Check sheet for the modelled part. Datum: model origin and axes. Units: mm. Face numbers are marked on the shaded views. A direction names the side the tool comes from. Round coordinates to 2 decimals unless told otherwise and drop trailing zeros. Write each loop counter-clockwise with the first axis right and the second up, starting at its lowest first coordinate (ties: lowest second). Pieces come first, ordered by that corner, then holes. Notation, with made-up numbers: (37.25, 59.25) -> (51.25, 59.25) arc R16 ccw to (51.25, 73.25) -> close; hole circle Ø9 at (-35, 39.25). An arc over 180 degrees is marked (long way). One line per item, written item: value.
from build123d import *

# Parameters (mm, degrees)
SKETCH1_W           = 38
SKETCH1_H           = 13
BOSS_EXTRUDE1_DEPTH = 65
SKETCH2_R           = 1.848381342
SKETCH2_R_2         = 4
SKETCH2_R_3         = 1.991530231
BOSS_EXTRUDE4_DEPTH = 22
SKETCH3_R           = 1.118624503
BOSS_EXTRUDE5_DEPTH = 15


with BuildPart() as part:
    # Sketch1 → Boss-Extrude1 (new body)
    with BuildSketch(Plane(origin=(0, 0, 0), x_dir=(0, 0, -1), z_dir=(1, 0, 0))):
        Rectangle(SKETCH1_W, SKETCH1_H)
    extrude(amount=BOSS_EXTRUDE1_DEPTH)

    # Sketch2 → Boss-Extrude4 (add)
    with BuildSketch(Plane(origin=(65, 0, 0), x_dir=(0, 0, -1), z_dir=(1, 0, 0))):
        with Locations(Location((-16.455259224, -3.564649458, 0), (0, 0, 180))):
            Circle(SKETCH2_R)
        with Locations(Location((-8.1, -2.100713402, 0), (0, 0, 180))):
            Circle(SKETCH2_R_2)
        with Locations(Location((0, -2.100713402, 0), (0, 0, 180))):
            Circle(SKETCH2_R_2)
        with Locations(Location((8.1, -2.100713402, 0), (0, 0, 180))):
            Circle(SKETCH2_R_2)
        with Locations(Location((16.444267151, -3.564649458, 0), (0, 0, 180))):
            Circle(SKETCH2_R_3)
    extrude(amount=BOSS_EXTRUDE4_DEPTH)

    # Sketch3 → Boss-Extrude5 (add)
    with BuildSketch(Plane.ZY):
        with Locations((-10.926639498, -2.758613366)):
            Circle(SKETCH3_R)
        with Locations((0, -2.758613366)):
            Circle(SKETCH3_R)
        with Locations((12.420208926, -2.758613366)):
            Circle(SKETCH3_R)
    extrude(amount=BOSS_EXTRUDE5_DEPTH)


solid = part.part
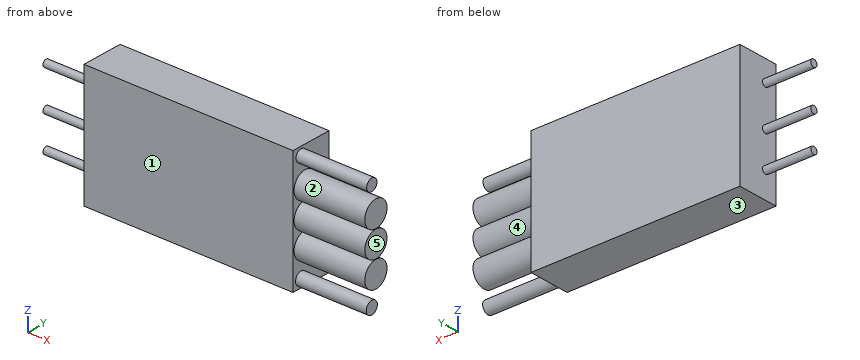
Item 1: Thickness scan on line 1 (X direction, y = -5.5, z = 15); line 2 (X direction, y = -3, z = 7); line 3 (Y direction, x = 66, z = -10). Record the ranges inside material, lowest first.
Answer:
line 1: x = 0 to 65
line 2: x = 0 to 87
line 3: y = -5.62 to 1.42
Item 2: Sectioned sample at C-C on z = 8.1. Enter the section's corners in (x, y), and give its area (3 significant figures).
Answer:
outline: (0, -6.5) -> (65, -6.5) -> (65, -6.1) -> (87, -6.1) -> (87, 1.9) -> (65, 1.9) -> (65, 6.5) -> (0, 6.5) -> close
area: 1,020 mm^2
Item 3: Mould release check, pull along Z, two halves, no side actions. Record for the marked faces 1, 2 and 3: pulls with the +Z half, pulls with the -Z half, needs draft (parallel to the pull), parting line crosses it, or undercut.
Answer:
face 1: needs draft
face 2: undercut
face 3: pulls with the -Z half
Item 4: Depth check by flat-ended pin: P1, Ø1.5, axis at y = -3, z = 9.5, coming from the -X side; P2, Ø5, axis at x = -1.5, y = -1, coming from the -Z side. Enter the tip coordinate at first touch or a pass-through.
Answer:
P1: stops at x = 0
P2: stops at z = -19
Item 5: Sectioned sample at B-B on x = 78. Enter the section's corners in (y, z), and give its area (3 significant figures).
Answer:
outline: circle Ø8 at (-2.1, -8.1); circle Ø8 at (-2.1, 0); circle Ø8 at (-2.1, 8.1); circle Ø3.98 at (-3.56, -16.44); circle Ø3.7 at (-3.56, 16.46)
area: 174 mm^2
Item 6: Tool access check on the marked faces 4 and 5. Record the directions out of +Z, -Z, +X, -X, +Y, -Y that give a thin tool (end or side, any length) a straight path to the whole face; none if there is none.
Answer:
face 4: +X
face 5: +Z, -Z, +X, +Y, -Y
Item 7: Sectioned sample at A-A on z = 0. Enter the section's corners in (x, y).
Answer:
outline: (-15, -3.88) -> (0, -3.88) -> (0, -6.5) -> (65, -6.5) -> (65, -6.1) -> (87, -6.1) -> (87, 1.9) -> (65, 1.9) -> (65, 6.5) -> (0, 6.5) -> (0, -1.64) -> (-15, -1.64) -> close
